```python
from build123d import *

# Parameters (mm, degrees)
F0_R     = 3.175
F1_DEPTH = 5.588
F2_R     = 1.27
F3_DEPTH = 15.24
F4_DEPTH = 19.05
F5_SIZE  = 1.27


with BuildPart() as f1:
    # F0 (on Front) → F1 (new body, symmetric)
    with BuildSketch(Plane.XZ):
        with BuildLine():
            ThreePointArc((32.5652864105, 5.461), (15.973258631, 28.8994015285), (-12.7, 30.48))
            Line((-12.7, 30.48), (-12.7, 13.97))
            ThreePointArc((-12.7, 13.97), (-14.5598719395, 9.4798719395), (-19.05, 7.62))
            Line((-19.05, 7.62), (-20.32, 7.62))
            Line((-20.32, 7.62), (-20.32, -7.62))
            Line((-20.32, -7.62), (-19.05, -7.62))
            ThreePointArc((-19.05, -7.62), (-14.5598719395, -9.4798719395), (-12.7, -13.97))
            Line((-12.7, -13.97), (-12.7, -30.48))
            ThreePointArc((-12.7, -30.48), (15.973258631, -28.8994015285), (32.5652864105, -5.461))
            ThreePointArc((32.5652864105, -5.461), (30.48, 0), (32.5652864105, 5.461))
        make_face()
        Circle(F0_R, mode=Mode.SUBTRACT)
    extrude(amount=F1_DEPTH, both=True)

    # F2 (on face) → F3 (cut)
    with BuildSketch(Plane(origin=(-20.32, 0, 0), x_dir=(0, -1, 0), z_dir=(-1, 0, 0))):
        Circle(F2_R)
        with Locations((0, 5.08)):
            Circle(F2_R)
        with Locations((0, -5.08)):
            Circle(F2_R)
    extrude(amount=-F3_DEPTH, mode=Mode.SUBTRACT)

    # F2 (on face) → F4 (cut)
    with BuildSketch(Plane(origin=(-20.32, 0, 0), x_dir=(0, -1, 0), z_dir=(-1, 0, 0))):
        Circle(F2_R)
    extrude(amount=-F4_DEPTH, mode=Mode.SUBTRACT)

    # F5
    f5_edges = [f1.edges().sort_by_distance(p)[0] for p in [
        (15.973259, -5.588, 28.899402),
        (15.973259, -5.588, -28.899402),
        (15.973259, 5.588, 28.899402),
        (15.973259, 5.588, -28.899402),
    ]]
    chamfer(f5_edges, length=F5_SIZE)


solid = f1.part
```
Source: CAD feature listing. Evaluate the final solid. Frame: model axes, mm. A direction names the side the tool comes from. Coordinates: 2 decimals unless noted, no trailing zeros. Loops run counter-clockwise (first coordinate to the right, second up) from the corner with the lowest first, then second, coordinate; pieces in that order, holes last. Notation, with made-up numbers: M 16.25,88 L 53.25,88 A14 cw 53.25,105 Z; hole C -13.5,12 d3. An arc over 180 degrees is marked long. Use a Markdown table: item, result. Add a question column.
Q1. Draft query along Y for faces 5 (the cylindrical face through (-14.61, -0.08, -9.43)), 6 (the cylindrical face through (-12.81, 0.17, -3.82)), 7 (the flat face through (-5.08, 0, -5)), 8 (the conical face through (15.433, -5.385, -27.978)). Return one class per face: pulls with the +Y half, pulls with the -Y half, needs draft (parallel to the pull), parting line crosses it, or undercut.
Q2. First-contact query: pin 1 (1 mm diameter, centred on y = 1.5, z = 24, fed in from -X); pin 2 (4 mm diameter, centred on x = 15, y = 3, fed in from -Z); pin 3 (0.6 mm diameter, centred on x = -20, y = -1, fed in from -Z). Flat tips, straight axial feed; report the tip coordinate or a pass-through.
Q3. Section query B-B, the plane x = 0. Return loops of the section in (y, z) (3 decimals).
Q4. Section query C-C, the plane z = -2. Return loops of the section in (x, y), and give its area (3 significant figures).
Q5. Material intervals for L1, parallel to Z at x = -15.5, y = 0; L2, parallel to Z at x = 0, y = 0 (3 decimals); L3, parallel to Z at x = -17.5, y = 1, sorted ascending.
Q6. Access query for faces 1 (the flat face through (-12.7, 0, 22)), 2 (the conical face through (16.155, 5.385, 27.568)), 3 (the flat face through (-12.7, 0, -22)), 4 (the cylindrical face through (-12.81, 0.28, 3.84)). Directions: +Z, -Z, +X, -X, +Y, -Y. A direction counts if a zero-diameter tool reaches every point of the face in a straight line with its end or side. Return the directions, or none.
Q7. Section query A-A, the plane y = 2.25. Return loops of the section in (x, z) (3 decimals), and give its area (3 significant figures).
Result:
| question | item | result |
|---|---|---|
| 1 | face 5 | needs draft |
| 1 | face 6 | undercut |
| 1 | face 7 | undercut |
| 1 | face 8 | pulls with the -Y half |
| 2 | pin 1 | stops at x = -12.7 |
| 2 | pin 2 | stops at z = -30.35 |
| 2 | pin 3 | stops at z = -7.62 |
| 3 | outline | M -5.588,-31.75 L -4.318,-33.02 L 4.318,-33.02 L 5.588,-31.75 L 5.588,-3.175 L -5.588,-3.175 Z; M -5.588,3.175 L 5.588,3.175 L 5.588,31.75 L 4.318,33.02 L -4.318,33.02 L -5.588,31.75 Z |
| 4 | outline | M -20.32,-5.59 L -2.47,-5.59 L -2.47,5.59 L -20.32,5.59 Z; M 2.47,-5.59 L 30.73,-5.59 L 30.73,5.59 L 2.47,5.59 Z |
| 4 | area | 515 mm2 |
| 5 | L1 | z = -8.71 to -6.35, -3.81 to -1.27, 1.27 to 3.81, 6.35 to 8.71 |
| 5 | L2 | z = -33.02 to -3.175, 3.175 to 33.02 |
| 5 | L3 | z = -7.81 to -5.86, -4.3 to -0.78, 0.78 to 4.3, 5.86 to 7.81 |
| 6 | face 1 | +Z, -X, +Y, -Y |
| 6 | face 2 | +Z, +Y |
| 6 | face 3 | -Z, -X, +Y, -Y |
| 6 | face 4 | -X |
| 7 | outline | M -20.32,-7.62 L -19.05,-7.62 A6.35 cw -12.7,-13.97 L -12.7,-30.48 A33.02 ccw 32.565,-5.461 A8.193 cw 32.565,5.461 A33.02 ccw -12.7,30.48 L -12.7,13.97 A6.35 cw -19.05,7.62 L -20.32,7.62 Z; hole C 0,0 d6.35 |
| 7 | area | 2,610 mm2 |
